Could you check a few things on this model? Use its own coordinates, in mm. Face numbers are marked on the shaded views. A direction names the side the tool comes from. Give positions to 0.01 mm unless a question says otherwise; leave off trailing zeros. Loops run counter-clockwise (first coordinate to the right, second up) from the corner with the lowest first, then second, coordinate; pieces in that order, holes last. Notation, with made-up numbers: (66.25, -39) -> (89.25, -39) arc R17 cw to (89.25, -33) -> close; hole circle Ø11 at (-9, 86.5). An arc over 180 degrees is marked (long way). Put each result on its own line as item: value.
```python
from build123d import *

# Parameters (mm, degrees)
SKETCH1_W           = 4.3
SKETCH1_H           = 15.2
BOSS_EXTRUDE1_DEPTH = 5
SKETCH2_W           = 2
SKETCH2_H           = 10.7
CUT_EXTRUDE1_DEPTH  = 2
SKETCH3_R           = 0.225
BOSS_EXTRUDE2_DEPTH = 4.3


with BuildPart() as part:
    # Sketch1 → Boss-Extrude1 (new body)
    with BuildSketch(Plane.XY):
        with Locations((2.15, 7.6)):
            Rectangle(SKETCH1_W, SKETCH1_H)
    extrude(amount=-BOSS_EXTRUDE1_DEPTH)

    # Sketch2 → Cut-Extrude1 (cut)
    with BuildSketch(Plane(origin=(4.3, 0, 0), x_dir=(0, 0, -1), z_dir=(1, 0, 0))):
        with Locations((2.5, 8.35)):
            Rectangle(SKETCH2_W, SKETCH2_H)
    extrude(amount=-CUT_EXTRUDE1_DEPTH, mode=Mode.SUBTRACT)

    # Sketch3 → Boss-Extrude2 (add)
    with BuildSketch(Plane.XZ):
        with Locations((1.23, -1.23)):
            Circle(SKETCH3_R)
        with Locations((1.23, -3.77)):
            Circle(SKETCH3_R)
        with Locations((3.2, -2.5)):
            Circle(SKETCH3_R)
    extrude(amount=BOSS_EXTRUDE2_DEPTH)


solid = part.part
```
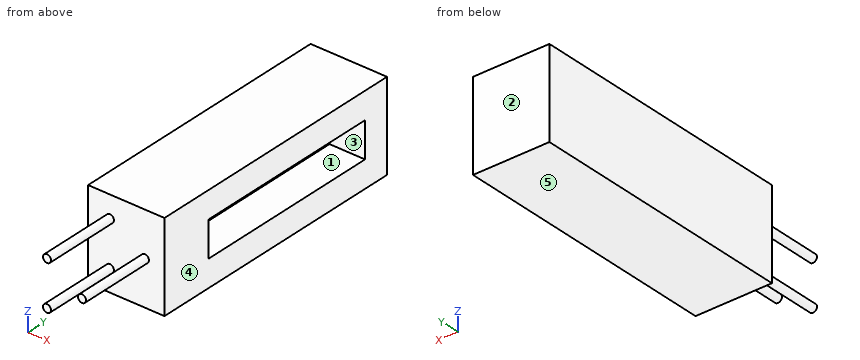
1. If we section it at D-D (x = 1.23): List the corners of the cut face in (y, z) for me (3 decimals), then the cut area to 3 significant figures.
Recorded:
outline: (-4.3, -3.995) -> (0, -3.995) -> (0, -5) -> (15.2, -5) -> (15.2, 0) -> (0, 0) -> (0, -1.005) -> (-4.3, -1.005) -> (-4.3, -1.455) -> (0, -1.455) -> (0, -3.545) -> (-4.3, -3.545) -> close
area: 79.9 mm^2
2. If we section it at A-A (z = -3.77): List the corners of the cut face in (x, y) for me (3 decimals), then the cut area to 3 significant figures.
Recorded:
outline: (0, 0) -> (1.005, 0) -> (1.005, -4.3) -> (1.455, -4.3) -> (1.455, 0) -> (4.3, 0) -> (4.3, 15.2) -> (0, 15.2) -> close
area: 67.3 mm^2
3. If we section it at C-C (x = 3.2): List the corners of the cut face in (y, z) for me (3 decimals).
Recorded:
outline: (-4.3, -2.725) -> (0, -2.725) -> (0, -5) -> (15.2, -5) -> (15.2, 0) -> (0, 0) -> (0, -2.275) -> (-4.3, -2.275) -> close; hole (3, -3.5) -> (13.7, -3.5) -> (13.7, -1.5) -> (3, -1.5) -> close
4. I need wall thicknesses on line 1 (Z direction, x = 3.8, y = 12); line 2 (Y direction, x = 3.2, z = -1.55); line 3 (Y direction, x = 0.6, z = -3.8). Which ranges of each line are inside material? Lowest first, please.
Recorded:
line 1: z = -5 to -3.5, -1.5 to 0
line 2: y = 0 to 3, 13.7 to 15.2
line 3: y = 0 to 15.2
5. Thinking about a two-plate mould opening in Z: for the marked faces 3, 4 and 5, which applies, pulls with the +Z half, pulls with the -Z half, needs draft (parallel to the pull), parting line crosses it, or undercut?
Recorded:
face 3: undercut
face 4: needs draft
face 5: pulls with the -Z half
6. For the marked faces 1 and 2, which set-ups out of +Z, -Z, +X, -X, +Y, -Y let a thin tool reach every point of the face, with its end or its side?
Recorded:
face 1: +X
face 2: +Z, -Z, +X, -X, +Y
7. I'm going to push flat-ended pins straight in: pin 1 (0.6 mm diameter, centred on x = 3, y = 6, fed in from +Z); pin 2 (0.6 mm diameter, centred on y = 10.5, z = -3, fed in from +X). Where does each tip first touch, or does it pass through?
Recorded:
pin 1: stops at z = 0
pin 2: stops at x = 2.3
8. If we section it at B-B (y = 9): List the corners of the cut face in (x, z) for me, then the cut area to 3 significant figures.
Recorded:
outline: (0, -5) -> (4.3, -5) -> (4.3, -3.5) -> (2.3, -3.5) -> (2.3, -1.5) -> (4.3, -1.5) -> (4.3, 0) -> (0, 0) -> close
area: 17.5 mm^2
